Geometry: see drawing. Coordinates: mm, zero at the bounding-box minimum. Coordinates: 2 decimals unless noted, no trailing zeros. Order: outer loops, then holes, each group sorted by start corner. A loop starts at its lowest first (then second) coordinate and runs counter-clockwise, first axis right, second up.
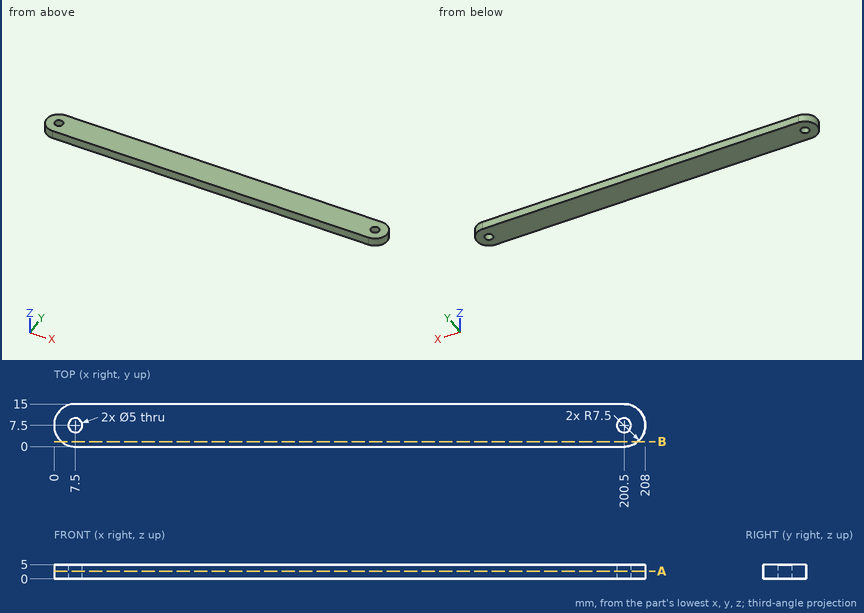
Item 1: Cut plane B-B on y = 1.75. Return loops of the section in (x, z).
Response values:
outline: (2.68, 0) - (205.32, 0) - (205.32, 5) - (2.68, 5) - close
Item 2: Ray query, probe 1 along X at (y, z) = (6.25, 1.9); probe 2 along Y at (x, z) = (200.5, 2.2); probe 3 along X at (y, z) = (12.5, 2.5). Return the intervals inside material, ascending.
Response values:
probe 1: x = 0.1 to 5.33, 9.67 to 198.33, 202.67 to 207.9
probe 2: y = 0 to 5, 10 to 15
probe 3: x = 1.91 to 206.09
Item 3: Pin query (flat end, axial travel): pin 1 Ø1 at (y, z) = (4.5, 4) entering from +X; pin 2 Ø2 at (y, z) = (2, 3.5) entering from -X; pin 3 Ø3 at (x, y) = (7.5, 7.5) entering from +Z. Return the tip coordinate at first contact, or that it passes through.
Response values:
pin 1: stops at x = 207.57
pin 2: stops at x = 1.5
pin 3: passes through
Item 4: Cut plane A-A on z = 2.7. Return loops of the section in (x, y), then the cut area to 3 significant figures.
Response values:
outline: (7.5, 0) - (200.5, 0) arc R7.5 ccw to (200.5, 15) - (7.5, 15) arc R7.5 ccw to start; hole circle Ø5 at (7.5, 7.5); hole circle Ø5 at (200.5, 7.5)
area: 3,030 mm2
